```python
from build123d import *

# Parameters (mm, degrees)
SKETCH_1_W          = 220
SKETCH_1_H          = 540
EXTRUDE_1_DEPTH     = 4
SKETCH_2_R          = 2.1
CUT_EXTRUDE_1_DEPTH = 292.575033225
SKETCH_4_R          = 93.8
CUT_EXTRUDE_2_DEPTH = 10
SKETCH_5_R          = 2.1
CUT_EXTRUDE_3_DEPTH = 10
SKETCH_6_R          = 1.7
SKETCH_6_R_2        = 1.65
CUT_EXTRUDE_5_DEPTH = 292.575033225


with BuildPart() as part:
    # 草图1 → 凸台-拉伸1 (new body)
    with BuildSketch(Plane.XY):
        Rectangle(SKETCH_1_W, SKETCH_1_H)
    extrude(amount=EXTRUDE_1_DEPTH)

    # 草图2 → 切除-拉伸1 (cut, through all)
    with BuildSketch(Plane(origin=(0, 0, 0), x_dir=(-1, 0, 0), z_dir=(0, 0, -1))):
        with Locations((100, -260)):
            Circle(SKETCH_2_R)
        with Locations((-100, -260)):
            Circle(SKETCH_2_R)
        with Locations(Location((100, 260, 0), (0, 0, 180))):
            Circle(SKETCH_2_R)
        with Locations(Location((-100, 260, 0), (0, 0, 180))):
            Circle(SKETCH_2_R)
        with Locations((-35, -260)):
            Circle(SKETCH_2_R)
        with Locations(Location((-35, 260, 0), (0, 0, 180))):
            Circle(SKETCH_2_R)
        with Locations((37.5, 260)):
            Circle(SKETCH_2_R)
        with Locations(Location((37.5, -260, 0), (0, 0, 180))):
            Circle(SKETCH_2_R)
    extrude(amount=-CUT_EXTRUDE_1_DEPTH, mode=Mode.SUBTRACT)

    # 草图4 → 切除-拉伸2 (cut)
    with BuildSketch(Plane.XY.offset(4)):
        with Locations((0, -45)):
            Circle(SKETCH_4_R)
    extrude(amount=-CUT_EXTRUDE_2_DEPTH, mode=Mode.SUBTRACT)

    # 草图5 → 切除-拉伸3 (cut)
    with BuildSketch(Plane.XY.offset(4)):
        with Locations((-100.25, 0)):
            Circle(SKETCH_5_R)
        with Locations((-70.887454814, 70.887454814)):
            Circle(SKETCH_5_R)
        with Locations((0, 100.25)):
            Circle(SKETCH_5_R)
        with Locations((70.887454814, 70.887454814)):
            Circle(SKETCH_5_R)
        with Locations((100.25, 0)):
            Circle(SKETCH_5_R)
        with Locations((70.887454814, -70.887454814)):
            Circle(SKETCH_5_R)
        with Locations((0, -100.25)):
            Circle(SKETCH_5_R)
        with Locations((-70.887454814, -70.887454814)):
            Circle(SKETCH_5_R)
        with Locations((-100.25, -125)):
            Circle(SKETCH_5_R)
        with Locations(Location((100.25, -125, 0), (0, 0, 180))):
            Circle(SKETCH_5_R)
        with Locations(Location((-100.25, 125, 0), (0, 0, 180))):
            Circle(SKETCH_5_R)
        with Locations((100.25, 125)):
            Circle(SKETCH_5_R)
    extrude(amount=-CUT_EXTRUDE_3_DEPTH, mode=Mode.SUBTRACT)

    # 草图6 → 切除-拉伸5 (cut, through all)
    with BuildSketch(Plane(origin=(0, 0, 0), x_dir=(-1, 0, 0), z_dir=(0, 0, -1))):
        with Locations((22.5, 240)):
            Circle(SKETCH_6_R)
        with Locations((-20, 240)):
            Circle(SKETCH_6_R)
        with Locations((22.5, 175.525642791)):
            Circle(SKETCH_6_R)
        with Locations((-20, 175.525642791)):
            Circle(SKETCH_6_R)
        with Locations((-35, 155.525642791)):
            Circle(SKETCH_6_R_2)
        with Locations((37.5, 155.525642791)):
            Circle(SKETCH_6_R_2)
    cut_extrude_5 = extrude(amount=-CUT_EXTRUDE_5_DEPTH, mode=Mode.SUBTRACT)

    # 镜向1: 切除-拉伸5 across plane
    add(cut_extrude_5.mirror(Plane.ZX), mode=Mode.SUBTRACT)


solid = part.part
```
Input: part model. Units: mm. Frame: model coordinates. Coordinates: 2 decimals unless noted, no trailing zeros. Order: outer loops, then holes, each group sorted by start corner. A loop starts at its lowest first (then second) coordinate and runs counter-clockwise, first axis right, second up. Notation, with made-up numbers: (12, 25) - (38, 25) arc R18 cw to (38, 30) - close; hole circle Ø9 at (28.25, -29). An arc over 180 degrees is marked (long way). Return JSON: item names as keys, results as strings.
Q1. Cut plane A-A (y = -86). Return loops of the section in (x, z), then the cut area to 3 significant figures.
The answers:
{"outline": "(-110, 0) - (-84.36, 0) - (-84.36, 4) - (-110, 4) - close; (84.36, 0) - (110, 0) - (110, 4) - (84.36, 4) - close", "area": "205 mm2"}
Q2. Cut plane B-B (x = -12). Return loops of the section in (y, z).
The answers:
{"outline": "(-270, 0) - (-138.03, 0) - (-138.03, 4) - (-270, 4) - close; (48.03, 0) - (270, 0) - (270, 4) - (48.03, 4) - close"}
Q3. Draft query along X for faces 1 (the flat face through (-2, 64, 4)), 2 (the cylindrical face through (89.47, -16.83, 2.03)). Return one class per face: +X half, -X half, draft (parallel to the pull), parting line (faces both ways), or undercut.
The answers:
{"face 1": "draft", "face 2": "undercut"}
Q4. Ray query, probe 1 along Y at (x, z) = (0, 1.5); probe 2 along X at (y, z) = (260, 2); probe 3 along Y at (x, z) = (-37.5, 2.1). Return the intervals inside material, ascending.
The answers:
{"probe 1": "y = -270 to -138.8, 48.8 to 98.15, 102.35 to 270", "probe 2": "x = -110 to -102.1, -97.9 to -39.6, -35.4 to 32.9, 37.1 to 97.9, 102.1 to 110", "probe 3": "y = -270 to -262.1, -257.9 to -157.18, -153.88 to -130.98, 40.98 to 153.88, 157.18 to 257.9, 262.1 to 270"}
Q5. Cut plane C-C (z = 2.25). State how many separate pieces and enclosed holes the cut face has, then the cut area to 3 significant figures.
The answers:
{"separate pieces": "1", "enclosed holes": "30", "area": "90,800 mm2"}
